Geometry check sheet. Reference: drawing and pictorial views, mm from the part's lowest x, y, z. A direction names the side the tool comes from. Round coordinates to 2 decimals unless told otherwise and drop trailing zeros. Write each loop counter-clockwise with the first axis right and the second up, starting at its lowest first coordinate (ties: lowest second). Pieces come first, ordered by that corner, then holes.
Item 1: Section check D-D, the plane y = 5.5. Record the cut outline in (x, z).
Item 2: Set-up check for the marked faces 4 and 5: record each of +Z, -Z, +X, -X, +Y, -Y from which the full face is reachable in a straight line by a thin tool's end or side.
Item 3: Depth check by flat-ended pin: pin 1 (5 mm diameter, centred on x = 33.5, y = 13.5, fed in from +Z); pin 2 (12 mm diameter, centred on x = 21.5, y = 36.5, fed in from -Z); pin 3 (1.5 mm diameter, centred on x = 65, z = 20, fed in from -Y); pin 4 (2 mm diameter, centred on y = 20.5, z = 0.5, fed in from -X). Enter the tip coordinate at first touch or a pass-through.
Item 4: Material ranges on line 1 along Y through (x, z) = (92.5, 0.7); line 2 along X through (y, z) = (48, 26); line 3 along Z through (x, y) = (13.5, 51.5), recorded low to high.
Item 5: Section check B-B, the plane y = 25. Record the cut outline in (x, z).
Item 6: Release check for a two-part mould opening along Z. For the marked faces 1, 2 and 3 record: pulls with the +Z half, pulls with the -Z half, needs draft (parallel to the pull), parting line crosses it, or undercut.
Item 7: Section check C-C, the plane x = 92.5. Record the cut outline in (y, z), plus the area to 3 significant figures.
Item 8: Section check A-A, the plane x = 17.5. Record the cut outline in (y, z), plus the area to 3 significant figures.
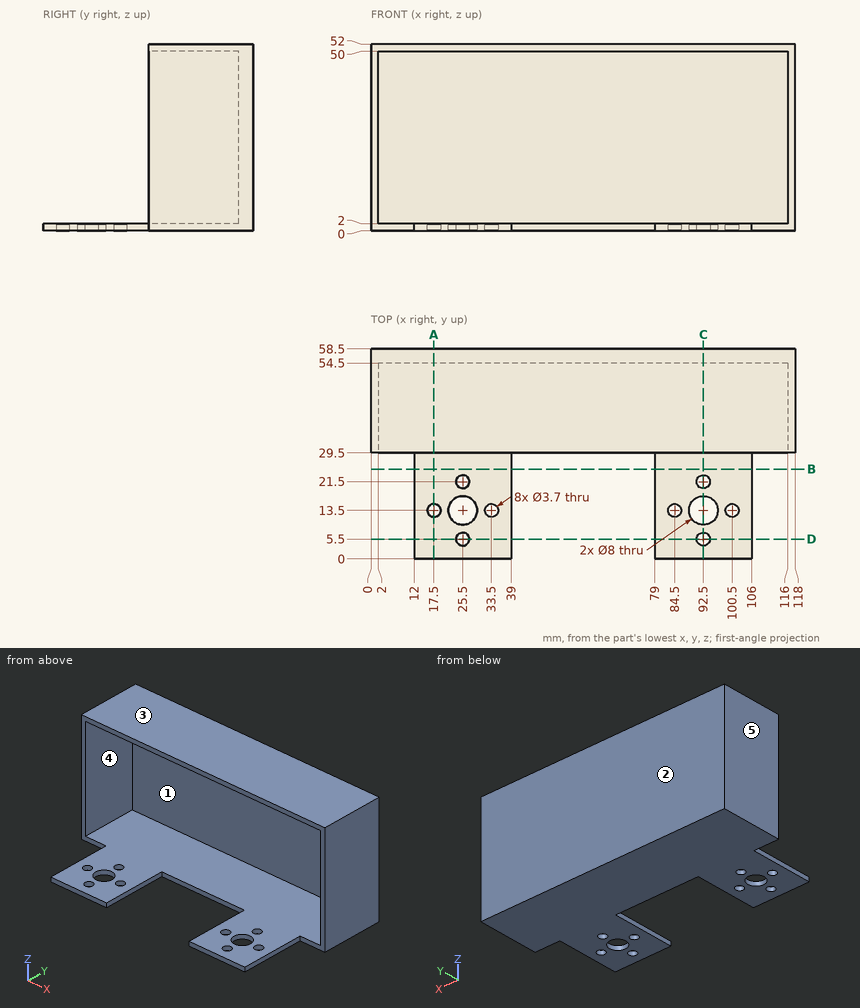
Values found:
1. outline: (12, 0) - (23.65, 0) - (23.65, 2) - (12, 2) - close; (27.35, 0) - (39, 0) - (39, 2) - (27.35, 2) - close; (79, 0) - (90.65, 0) - (90.65, 2) - (79, 2) - close; (94.35, 0) - (106, 0) - (106, 2) - (94.35, 2) - close
2. face 4: -Y
2. face 5: +Z, -Z, -X, +Y, -Y
3. pin 1: stops at z = 2
3. pin 2: stops at z = 0
3. pin 3: stops at y = 54.5
3. pin 4: stops at x = 12
4. line 1: y = 0 to 3.65, 7.35 to 9.5, 17.5 to 19.65, 23.35 to 58.5
4. line 2: x = 0 to 2, 116 to 118
4. line 3: z = 0 to 2, 50 to 52
5. outline: (12, 0) - (39, 0) - (39, 2) - (12, 2) - close; (79, 0) - (106, 0) - (106, 2) - (79, 2) - close
6. face 1: undercut
6. face 2: needs draft
6. face 3: pulls with the +Z half
7. outline: (0, 0) - (3.65, 0) - (3.65, 2) - (0, 2) - close; (7.35, 0) - (9.5, 0) - (9.5, 2) - (7.35, 2) - close; (17.5, 0) - (19.65, 0) - (19.65, 2) - (17.5, 2) - close; (23.35, 0) - (58.5, 0) - (58.5, 52) - (29.5, 52) - (29.5, 50) - (54.5, 50) - (54.5, 2) - (23.35, 2) - close
7. area: 336 mm2
8. outline: (0, 0) - (11.65, 0) - (11.65, 2) - (0, 2) - close; (15.35, 0) - (58.5, 0) - (58.5, 52) - (29.5, 52) - (29.5, 50) - (54.5, 50) - (54.5, 2) - (15.35, 2) - close
8. area: 360 mm2
